Can you work these out from the drawing? Everything is in mm from the part's minimum corner. A direction names the side the tool comes from. Give positions to 0.01 mm unless a question says otherwise; leave off trailing zeros. Loops run counter-clockwise (first coordinate to the right, second up) from the corner with the lowest first, then second, coordinate; pieces in that order, holes last.
Q1. I need wall thicknesses on line 1 (X direction, y = 2, z = 2.5); line 2 (Y direction, x = 3.5, z = 3.5); line 3 (Y direction, x = 1, z = 5). Which ranges of each line are inside material? Lowest first, please.
Q2. Will these pins go through, and if not, where does the flat tip stop? P1, Ø0.8, axis at x = 4, z = 0.5, coming from the +Y side; P2, Ø1.5, axis at x = 3, y = 6, coming from the +Z side; P3, Ø0.8, axis at x = 0.5, y = 6, coming from the +Z side.
Q3. If we section it at D-D (y = 4.5): Please give me the cut outline in (x, z), plus the area to 3 significant figures.
Q4. If we section it at C-C (z = 3.5): Please give me the cut outline in (x, y).
Q5. For the marked faces 4, 5, 6 and 7, which set-ups out of +Z, -Z, +X, -X, +Y, -Y let a thin tool reach every point of the face, with its end or its side?
Q6. We'd pull the mould along X, two halves only. Please class the marked faces 1, 2 and 3: +X half, -X half, draft (parallel to the pull), parting line (faces both ways), or undercut.
Q7. If we section it at B-B (x = 6.25): Please give me the cut outline in (y, z).
Q8. If we section it at A-A (y = 2.25): Please give me the cut outline in (x, z).
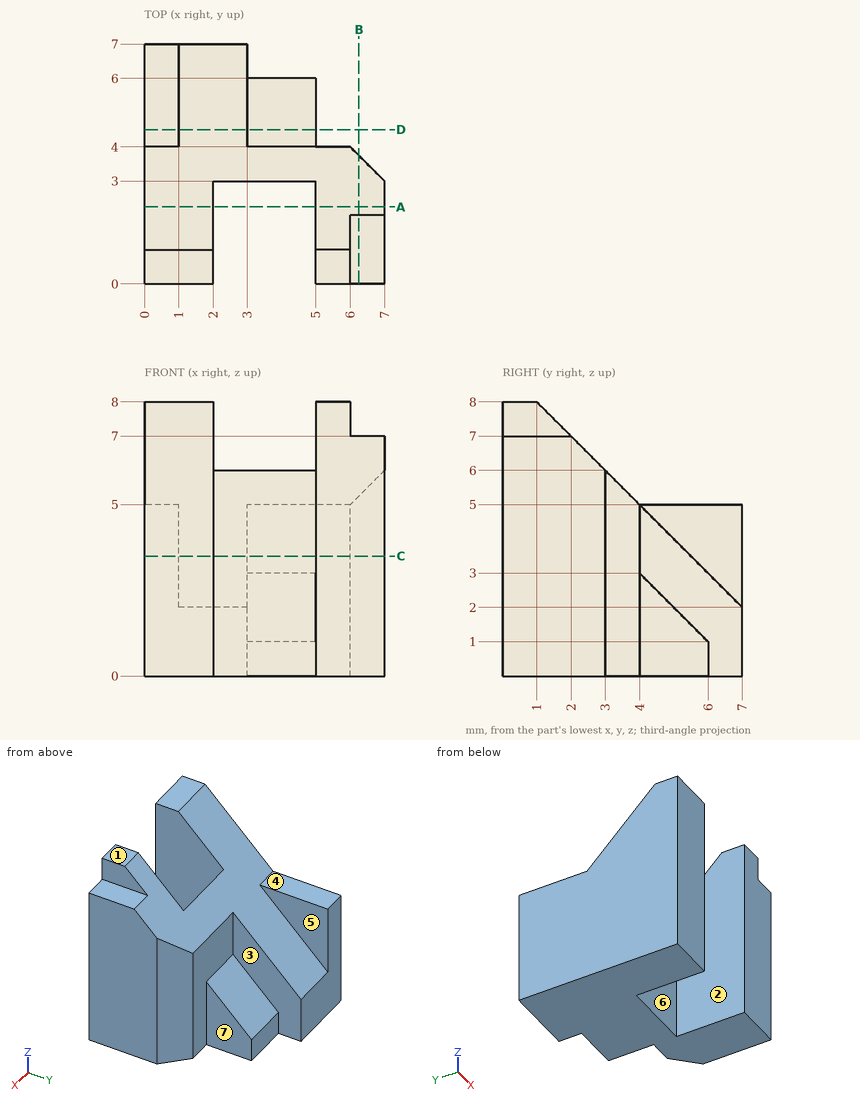
Check sheet entries:
1. line 1: x = 0 to 2, 5 to 7
1. line 2: y = 3 to 4
1. line 3: y = 0 to 4
2. P1: stops at y = 6
2. P2: stops at z = 3.75
2. P3: stops at z = 5
3. outline: (0, 0) - (5, 0) - (5, 2.5) - (3, 2.5) - (3, 4.5) - (1, 4.5) - (1, 5) - (0, 5) - close
3. area: 19.0 mm2
4. outline: (0, 0) - (2, 0) - (2, 3) - (5, 3) - (5, 0) - (7, 0) - (7, 3) - (6, 4) - (3, 4) - (3, 5.5) - (1, 5.5) - (1, 7) - (0, 7) - close
5. face 4: +Z, +X, -X, +Y
5. face 5: +Z, +X, +Y
5. face 6: +Z, -Z, -Y
5. face 7: +Z, -Z, +X, +Y
6. face 1: draft
6. face 2: undercut
6. face 3: +X half
7. outline: (0, 0) - (3.75, 0) - (3.75, 5.25) - (2, 7) - (0, 7) - close
8. outline: (0, 0) - (2, 0) - (2, 6.75) - (0, 6.75) - close; (5, 0) - (7, 0) - (7, 6.75) - (5, 6.75) - close
